Check sheet for the modelled part. Datum: model origin and axes. Units: mm. Coordinates: 2 decimals unless noted, no trailing zeros. Loops run counter-clockwise (first coordinate to the right, second up) from the corner with the lowest first, then second, coordinate; pieces in that order, holes last.
Autodesk Inventor part; units mm, degrees
ref_plane "YZ Plane" through (0, 0, 0) normal (1, 0, 0) x (0, 1, 0)
ref_plane "XZ Plane" through (0, 0, 0) normal (0, 1, 0) x (-1, 0, 0)
ref_plane "XY Plane" through (0, 0, 0) normal (0, 0, 1) x (1, 0, 0)
sketch "Sketch1" plane through (0, 0, 0) normal (0, 0, 1) x (1, 0, 0)
  circle A0 centre (0, 0) radius 3.175
  circle A1 centre (0, 0) radius 6.35
  dimension "d0" = 6.35
  dimension "d1" = 12.7
extrude "Extrusion1" add sketch "Sketch1" against normal blind 12.7
chamfer "Chamfer1" distance 3.175 angle 45 2 edges at (-6.35, 0, 0) (-6.35, 0, -12.7)
fillet "Fillet1" radius 3.175 2 edges at (-6.35, 0, -3.1745) (-6.35, 0, -9.5255)
properties part number "Handle" material "Aluminum 6061"
1) Depth check by flat-ended pin: pin 1 (6 mm diameter, centred on y = -4.5, z = -7.5, fed in from -X); pin 2 (1 mm diameter, centred on x = 4.5, y = -0.5, fed in from -Z); pin 3 (1.5 mm diameter, centred on y = 1, z = -5.5, fed in from -X). Enter the tip coordinate at first touch or a pass-through.
Answer sheet:
pin 1: stops at x = -6.17
pin 2: stops at z = -11.85
pin 3: stops at x = -6.35
2) Section check A-A on z = -4.75. Enter the section's corners in (x, y) (3 decimals), plus the area to 3 significant figures.
Answer sheet:
outline: circle Ø12.7 at (0, 0); hole circle Ø6.35 at (0, 0)
area: 95.0 mm2
3) Scan lines: line 1 (Y direction, x = 0, z = -6.25) (3 decimals); line 2 (Y direction, x = 0, z = -10) (3 decimals); line 3 (X direction, y = -1.75, z = -4). Record each from-to range of solid material in increasing order.
Answer sheet:
line 1: y = -6.35 to -3.175, 3.175 to 6.35
line 2: y = -5.798 to -3.175, 3.175 to 5.798
line 3: x = -6.06 to -2.65, 2.65 to 6.06
4) Mould release check, pull along Y, two halves, no side actions. Record for faces 1 (the cylindrical face through (-1.38, -6.2, -6.32)), 2 (the cylindrical face through (-0.69, -3.1, -6.26)): +Y half, -Y half, draft (parallel to the pull), parting line (faces both ways), or undercut.
Answer sheet:
face 1: parting line
face 2: undercut
